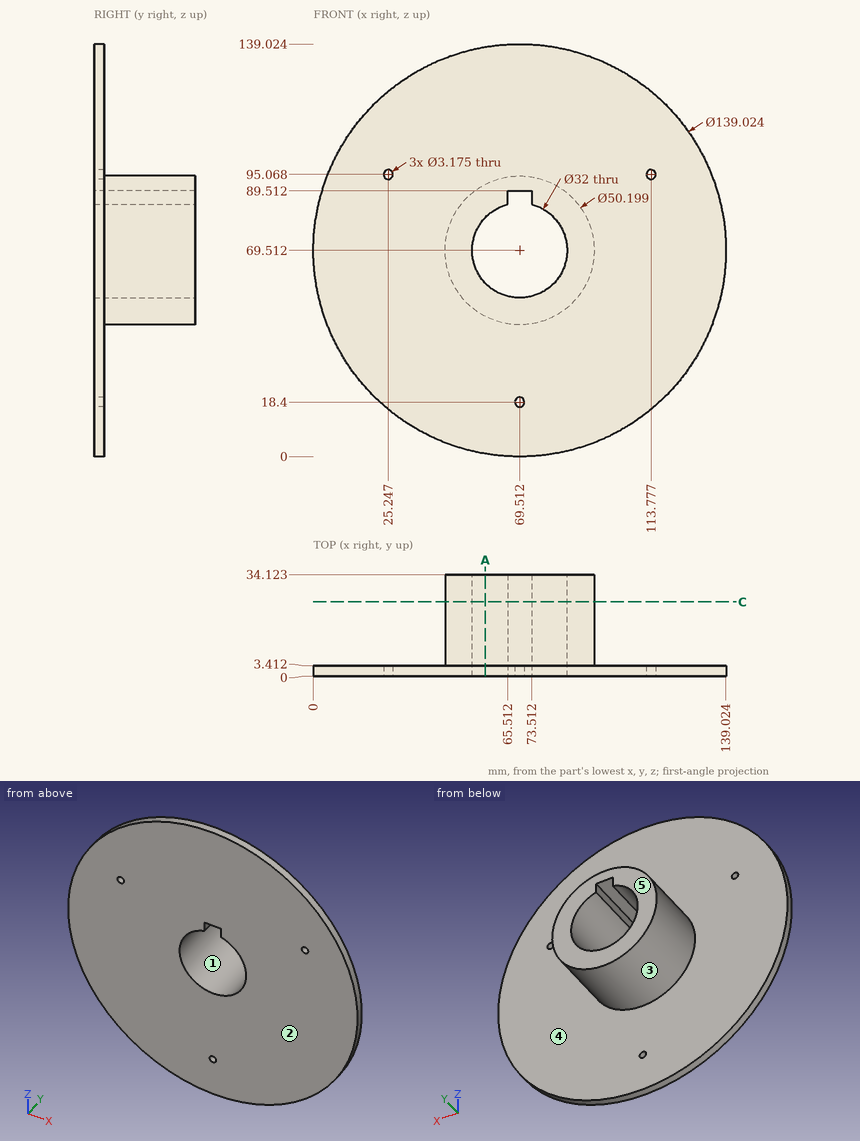
Geometry: see drawing. Coordinates: mm, zero at the bounding-box minimum. A direction names the side the tool comes from. Coordinates: 2 decimals unless noted, no trailing zeros. Order: outer loops, then holes, each group sorted by start corner. A loop starts at its lowest first (then second) coordinate and runs counter-clockwise, first axis right, second up. Notation, with made-up numbers: M 9,62 L 33,62 A21 ccw 33,88 Z; hole C 54,24.25 d7. An arc over 180 degrees is marked long. Write each question's results on one line, items separated by ' | '. Start each with the question number.
1) Access query for the marked faces 4 and 5. Directions: +Z, -Z, +X, -X, +Y, -Y. A direction counts if a zero-diameter tool reaches every point of the face in a straight line with its end or side. Return the directions, or none.
2) Draft query along Z for the marked faces 1, 2 and 3. Return one class per face: released by +Z, released by -Z, zero draft, split by the parting line, or undercut.
3) Contact query for flat-ended pins moving along their axis: pin 1 Ø4 at (x, y) = (83, 27.5) entering from +Z; pin 2 Ø1 at (x, y) = (50, 26.5) entering from -Z (1 decimal); pin 3 Ø2.5 at (x, z) = (69.51, 18.4) entering from +Y; pin 4 Ø2.5 at (x, y) = (71, 18) entering from -Z. Output: stop coordinate, or through.
4) Section query A-A (x = 58). Return the cut outline in (y, z) (1 decimal).
5) Line query: line 1 (Y direction, x = 12, z = 75.5); line 2 (X direction, y = 14.5, z = 86.5) (1 decimal); line 3 (X direction, y = 11, z = 62) (1 decimal). Output: solid intervals per line, ascending. Write a range as from..to.
6) Section query C-C (y = 25). Return the cut outline in (x, z).
Answers:
1) face 4: +Y | face 5: +Z, -Z, +X, -X, +Y
2) face 1: undercut | face 2: zero draft | face 3: split by the parting line
3) pin 1: stops at z = 91.83 | pin 2: stops at z = 53.1 | pin 3: passes through | pin 4: stops at z = 44.41
4) outline: M 0,1 L 3.4,1 L 3.4,47.2 L 34.1,47.2 L 34.1,58.4 L 0,58.4 Z; M 0,80.6 L 34.1,80.6 L 34.1,91.8 L 3.4,91.8 L 3.4,138.1 L 0,138.1 Z
5) line 1: y = 0..3.41 | line 2: x = 51..65.5, 73.5..88 | line 3: x = 45.6..55.4, 83.6..93.5
6) outline: C 69.51,69.51 d50.2; hole M 65.51,85 A16 ccw long 73.51,85 L 73.51,89.51 L 65.51,89.51 Z
